The listing builds one solid part. Answer for the finished solid, in the listing's coordinates (mm). Coordinates: 2 decimals unless noted, no trailing zeros. Order: outer loops, then holes, each group sorted by start corner. A loop starts at its lowest first (then second) coordinate and runs counter-clockwise, first axis right, second up. Notation, with made-up numbers: M -7.5,28 L 40.5,28 A14 cw 40.5,34 Z; hole C 55.25,10.25 d9. An arc over 180 degrees is marked long. One line per item, written item: value. Start each with the question number.
Q1. The part is cut by section C-C on z = 4.5. Give the vertices of the cut face in (x, y), then the cut area to 3 significant figures.
Q2. The part is cut by section B-B on y = 35. Give the vertices of the cut face in (x, z), then the cut area to 3 significant figures.
Q3. This flat-tipped pin is pushed along its axis until it touches: pin 1 Ø5 at (x, y) = (11.43, 34.29) entering from -Z. Where does it stop, or does it pass through?
Q4. Straight lines are drawn through the part: line 1 along Y through (x, z) = (4.5, 5.5); line 2 along Y through (x, z) = (11.43, 2); line 3 along Y through (x, z) = (14, 3.5). For each, find the intervals that lie inside material, in ascending order. Write a range as [from, to].
Q5. The part is cut by section A-A on x = 11.43. Give the vertices of the cut face in (y, z), then the cut area to 3 significant figures.
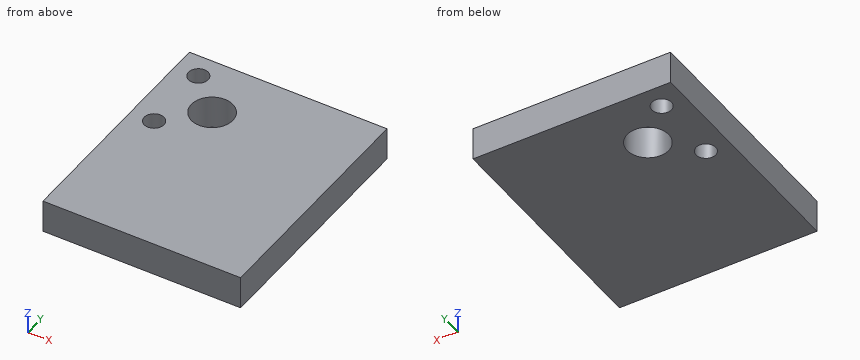
```python
from build123d import *

# Parameters (mm, degrees)
SKETCH1_W                 = 38.1
SKETCH1_H                 = 45.72
BOSS_EXTRUDE1_DEPTH       = 6.35
SKETCH2_R                 = 4
CUT_EXTRUDE1_DEPTH        = 1
CUT_EXTRUDE1_DEPTH_BACK   = 7.35
F_6_CLEARANCE_HOLE2_D     = 3.7973
F_6_CLEARANCE_HOLE2_DEPTH = 6.35


with BuildPart() as part:
    # Sketch1 → Boss-Extrude1 (new body)
    with BuildSketch(Plane.XY):
        with Locations((19.05, 22.86)):
            Rectangle(SKETCH1_W, SKETCH1_H)
    extrude(amount=BOSS_EXTRUDE1_DEPTH)

    # Sketch2 → Cut-Extrude1 (cut, two sides)
    with BuildSketch(Plane.XY.offset(6.35)) as cut_extrude1_sk:
        with Locations((11.43, 34.29)):
            Circle(SKETCH2_R)
    extrude(amount=CUT_EXTRUDE1_DEPTH, mode=Mode.SUBTRACT)
    extrude(cut_extrude1_sk.sketch, amount=-CUT_EXTRUDE1_DEPTH_BACK, mode=Mode.SUBTRACT)

    # #6 Clearance Hole2
    with Locations(Plane.XY.offset(6.35)):
        with Locations((4.515202787, 41.204797213), (4.515202787, 27.375202787)):
            Hole(F_6_CLEARANCE_HOLE2_D / 2, depth=F_6_CLEARANCE_HOLE2_DEPTH)


solid = part.part
```
Output:
1. outline: M 0,0 L 38.1,0 L 38.1,45.72 L 0,45.72 Z; hole C 4.52,27.38 d3.8; hole C 4.52,41.2 d3.8; hole C 11.43,34.29 d8
1. area: 1,670 mm^2
2. outline: M 0,0 L 7.49,0 L 7.49,6.35 L 0,6.35 Z; M 15.37,0 L 38.1,0 L 38.1,6.35 L 15.37,6.35 Z
2. area: 192 mm^2
3. pin 1: passes through
4. line 1: y = [0, 25.48], [29.27, 39.31], [43.1, 45.72]
4. line 2: y = [0, 30.29], [38.29, 45.72]
4. line 3: y = [0, 31.22], [37.36, 45.72]
5. outline: M 0,0 L 30.29,0 L 30.29,6.35 L 0,6.35 Z; M 38.29,0 L 45.72,0 L 45.72,6.35 L 38.29,6.35 Z
5. area: 240 mm^2
